Design review of the part shown in the three views and the two pictorial views. Dimensions are in mm from the part's minimum x, y and z. A direction names the side the tool comes from. Give positions to 0.01 mm unless a question says otherwise; leave off trailing zeros. Loops run counter-clockwise (first coordinate to the right, second up) from the corner with the lowest first, then second, coordinate; pieces in that order, holes last. Notation, with made-up numbers: (88, 44.5) - (138, 44.5) arc R14 ccw to (138, 51.5) - close; hole circle Ø3 at (59.5, 65). An arc over 180 degrees is marked (long way). Use CSV: the item, a comma, the result in double quotes. Start each with the question number.
1. Mouldability with a two-part tool opening along Z and no side actions: class the marked faces 4, 5 and 6 as pulls with the +Z half, pulls with the -Z half, needs draft (parallel to the pull), parting line crosses it, or undercut.
2. Take a section at D-D on x = 62. Give the boundary of the cut face in (y, z), plus the area to 3 significant figures.
3. For the marked faces 1, 2 and 3, list the 3-axis set-ups (+Z, -Z, +X, -X, +Y, -Y) from which the entire face can be reached by the end or side of a thin tool; tool diameter is ignored.
4. For pin 1 (3 mm diameter, centred on x = 14.5, z = 25, fed in from +Y); pin 2 (7 mm diameter, centred on x = 15.5, y = 2, fed in from -Z) (1 decimal); pin 3 (5 mm diameter, centred on x = 12.5, y = 4, fed in from +Z) (1 decimal), all flat-tipped, find the tip position at first contact; note any pin that passes through.
5. Wall thickness on line 1 (Y direction, x = 14, z = 56); line 2 (X direction, y = 11.5, z = 36.5) (1 decimal); line 3 (X direction, y = 2.5, z = 38) (1 decimal): over which ranges is each line inside the solid? List them lowest first.
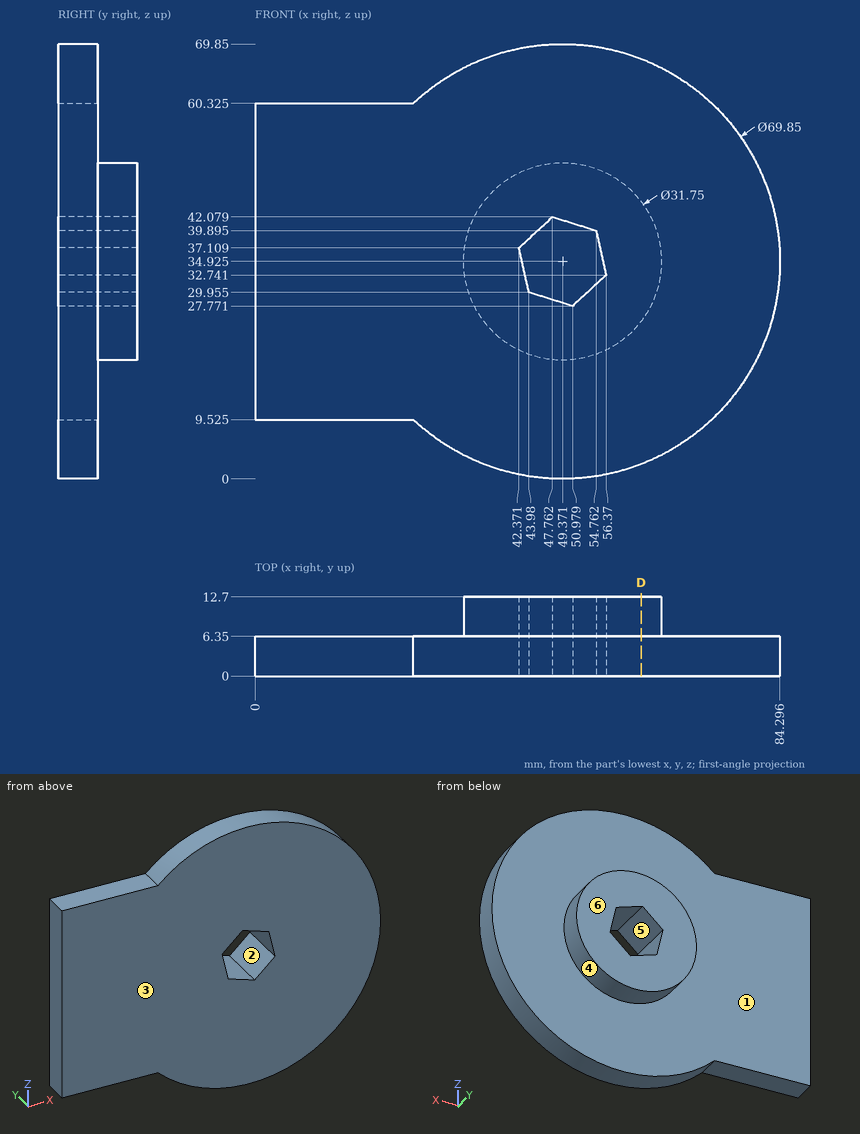
Check result:
1,face 4,"parting line crosses it"
1,face 5,"undercut"
1,face 6,"needs draft"
2,outline,"(0, 2.36) - (6.35, 2.36) - (6.35, 25.31) - (12.7, 25.31) - (12.7, 44.54) - (6.35, 44.54) - (6.35, 67.49) - (0, 67.49) - close"
2,area,"536 mm²"
3,face 1,"+Y"
3,face 2,"+Y, -Y"
3,face 3,"+Z, -Z, +X, -X, -Y"
4,pin 1,"stops at y = 6.35"
4,pin 2,"stops at z = 9.5"
4,pin 3,"stops at z = 60.3"
5,line 1,"y = 0 to 6.35"
5,line 2,"x = 33.6 to 42.5, 55.5 to 65.2"
5,line 3,"x = 0 to 43.3, 55.2 to 84.2"
